Design review of the part built by this model. Coordinates are the model's own, in mm. A direction names the side the tool comes from. Round coordinates to 2 decimals unless told otherwise and drop trailing zeros. Loops run counter-clockwise (first coordinate to the right, second up) from the corner with the lowest first, then second, coordinate; pieces in that order, holes last. Notation, with made-up numbers: (43.25, 77) -> (97.25, 77) arc R30 cw to (97.25, 99) -> close; hole circle Ø11 at (0, 85.5). An arc over 180 degrees is marked (long way). Answer as CSV lines item,"result". Start each with the question number.
(1) For P1, Ø1.2, axis at x = 2.5, z = -1, coming from the +Y side; P2, Ø1.2, axis at x = 3, z = -0.5, coming from the -Y side; P3, Ø1.6, axis at y = 4.5, z = -0.5, coming from the +X side, all flat-tipped, find the tip position at first contact; note any pin that passes through.
(2) To check wall thickness, follow line 1 (Y direction, x = 3.75, z = -1.25); line 2 (Z direction, x = 0.5, y = 3.75); line 3 (Z direction, x = -0.25, y = 5.25). State the ranges of each line that lie inside material, in increasing order. Write a range as from..to.
(3) Machinability: for faces 1 (the face through (4.173, 4.783, 1.479)), 2 (the face through (3, 6, -1)), 3 (the face through (6, 3, -1)), which of the approach directions +Z, -Z, +X, -X, +Y, -Y give a long, thin tool a straight path to every point of the face, cutting with its end or side? Answer none if there is none.
(4) Take a section at D-D, the plane x = 3. Write out the cut boundary in (y, z), and give its area (3 significant figures).
(5) Take a section at A-A, the plane x = 0.25. Write out the cut boundary in (y, z).
(6) Take a section at C-C, the plane z = -0.75. Write out the cut boundary in (x, y), and give its area (3 significant figures).
from build123d import *

# Parameters (mm, degrees)
SKETCH1_W           = 6
SKETCH1_H           = 6
BOSS_EXTRUDE1_DEPTH = 1.5
SKETCH2_R           = 2.181214146
BOSS_EXTRUDE2_DEPTH = 3
SKETCH4_W           = 8
SKETCH4_H           = 8
BOSS_EXTRUDE3_DEPTH = 3


with BuildPart() as part:
    # Sketch1 → Boss-Extrude1 (new body)
    with BuildSketch(Plane.XY):
        with Locations((3, 3)):
            Rectangle(SKETCH1_W, SKETCH1_H)
    extrude(amount=-BOSS_EXTRUDE1_DEPTH)

    # Sketch2 → Boss-Extrude2 (add)
    with BuildSketch(Plane.XY):
        with Locations((3, 2.94366618)):
            Circle(SKETCH2_R)
    extrude(amount=BOSS_EXTRUDE2_DEPTH)

    # Sketch4 → Boss-Extrude3 (add)
    with BuildSketch(Plane(origin=(0, 0, -1.5), x_dir=(-1, 0, 0), z_dir=(0, 0, -1))):
        with Locations((-3, 3)):
            Rectangle(SKETCH4_W, SKETCH4_H)
    extrude(amount=BOSS_EXTRUDE3_DEPTH)


solid = part.part
The answers:
1,P1,"y = 7"
1,P2,"y = 0"
1,P3,"x = 6"
2,line 1,"0..6"
2,line 2,"-4.5..0"
2,line 3,"-4.5..-1.5"
3,face 1,"+Z"
3,face 2,"+Z, +X, -X, +Y"
3,face 3,"+Z, +X, +Y, -Y"
4,outline,"(-1, -4.5) -> (7, -4.5) -> (7, -1.5) -> (6, -1.5) -> (6, 0) -> (5.12, 0) -> (5.12, 3) -> (0.76, 3) -> (0.76, 0) -> (0, 0) -> (0, -1.5) -> (-1, -1.5) -> close"
4,area,"46.1 mm²"
5,outline,"(-1, -4.5) -> (7, -4.5) -> (7, -1.5) -> (6, -1.5) -> (6, 0) -> (0, 0) -> (0, -1.5) -> (-1, -1.5) -> close"
6,outline,"(0, 0) -> (6, 0) -> (6, 6) -> (0, 6) -> close"
6,area,"36.0 mm²"
